Read the model definition and answer for the solid it produces. Units are mm, in the model's axes. A direction names the side the tool comes from. Give positions to 0.01 mm unless a question says otherwise; leave off trailing zeros. Order: outer loops, then holes, each group sorted by start corner. A loop starts at its lowest first (then second) coordinate and runs counter-clockwise, first axis right, second up. Notation, with made-up numbers: (49.25, 29.25) - (89.25, 29.25) arc R27 ccw to (89.25, 66.25) - close; hole circle Ø1 at (27, 53.25). An arc over 180 degrees is marked (long way). Return JSON: item names as keys, results as strings.
```python
from build123d import *

# Parameters (mm, degrees)
F0_R       = 29.175
F1_DEPTH   = 8.35
F1_FACE_R  = 29.175
F3_R       = 15.685
F5_R       = 15.685
F6_DEPTH   = 2.25
F7_R       = 16.25
F8_DEPTH   = 5.75
F9_R       = 29.625
F10_DEPTH  = 14.2
F11_R      = 21
F12_DEPTH  = 8.75
F12_FACE_R = 21
F14_R      = 35
F16_R      = 35
F17_DEPTH  = 10


with BuildPart() as f1:
    # F0 (on Top) → F1 (new body)
    with BuildSketch(Plane.XY):
        Circle(F0_R)
    extrude(amount=F1_DEPTH)

    # F1_face (on face) → F4 section 0
    with BuildSketch(Plane(origin=(0, 0, 0), x_dir=(1, 0, 0), z_dir=(0, 0, -1))):
        Circle(F1_FACE_R)
    # F3 (on offset) → F4 section 1
    with BuildSketch(Plane(origin=(0, 0, -18), x_dir=(1, 0, 0), z_dir=(0, 0, -1))):
        Circle(F3_R)
    loft()

    # F5 (on face) → F6 (join)
    with BuildSketch(Plane(origin=(0, 0, -18), x_dir=(1, 0, 0), z_dir=(0, 0, -1))):
        Circle(F5_R)
    extrude(amount=F6_DEPTH)

    # F7 (on face) → F8 (join)
    with BuildSketch(Plane(origin=(0, 0, -20.25), x_dir=(1, 0, 0), z_dir=(0, 0, -1))):
        Circle(F7_R)
    extrude(amount=F8_DEPTH)

    # F9 (on face) → F10 (join)
    with BuildSketch(Plane(origin=(0, 0, -26), x_dir=(1, 0, 0), z_dir=(0, 0, -1))):
        Circle(F9_R)
    extrude(amount=F10_DEPTH)

    # F11 (on face) → F12 (join)
    with BuildSketch(Plane(origin=(0, 0, -40.2), x_dir=(1, 0, 0), z_dir=(0, 0, -1))):
        Circle(F11_R)
    extrude(amount=F12_DEPTH)

    # F12_face (on face) → F15 section 0
    with BuildSketch(Plane(origin=(0, 0, -48.95), x_dir=(1, 0, 0), z_dir=(0, 0, -1))):
        Circle(F12_FACE_R)
    # F14 (on offset) → F15 section 1
    with BuildSketch(Plane(origin=(0, 0, -63.45), x_dir=(1, 0, 0), z_dir=(0, 0, -1))):
        Circle(F14_R)
    loft()

    # F16 (on face) → F17 (join)
    with BuildSketch(Plane(origin=(0, 0, -63.45), x_dir=(1, 0, 0), z_dir=(0, 0, -1))):
        Circle(F16_R)
    extrude(amount=F17_DEPTH)


solid = f1.part
```
Q1. Consider L1, parallel to Z at x = 3.5, y = 25; L2, parallel to Z at x = -16.5, y = -3; L3, parallel to Z at x = -8.5, y = 14. Determine where each line is inside the solid, lowest interval first.
Values:
{"L1": "z = -73.45 to -53.35, -40.2 to -26, -5.25 to 8.35", "L2": "z = -73.45 to -26, -16.55 to 8.35", "L3": "z = -73.45 to -26, -17.07 to 8.35"}
Q2. Determine the mould class of faces 1 (the conical face through (20.9, -6.6, -49.9)), 2 (the flat face through (0, 0, -73.45)), 3 (the cylindrical face through (-28, 21, -68)), 4 (the flat face through (13, 13, -26)) for opening direction Z: released by +Z, released by -Z, zero draft, split by the parting line, or undercut.
Values:
{"face 1": "undercut", "face 2": "released by -Z", "face 3": "zero draft", "face 4": "undercut"}
Q3. For faces 5 (the flat face through (-16, -1, -20.25)), 6 (the cylindrical face through (-6.325, -28.481, 4.117)), 7 (the flat face through (0, 0, 8.35)), determine the directions among +Z, -Z, +X, -X, +Y, -Y from which every point of the face is accessible in a straight line to the end or side of a thin tool.
Values:
{"face 5": "none", "face 6": "+Z", "face 7": "+Z, +X, -X, +Y, -Y"}
Q4. A cutting plane is placed at C-C (y = 27.5). Give the number of separate pieces and of enclosed holes in the cut face, and give its area (3 significant figures).
Values:
{"separate pieces": "3", "enclosed holes": "0", "area": "1,160 mm²"}
Q5. A cutting plane is placed at B-B (z = -47). Write down the section's boundary in (x, y).
Values:
{"outline": "circle Ø42 at (0, 0)"}
Q6. Given pin 1 (1 mm diameter, centred on x = 6.5, z = -13, fed in from -Y); pin 2 (10 mm diameter, centred on y = 24, z = -62, fed in from +X); pin 3 (8 mm diameter, centred on x = 9.5, z = -27, fed in from +Y), each flat-ended and moving along its own axis, determine where each tip first touches the part or whether it passes through.
Values:
{"pin 1": "stops at y = -18.75", "pin 2": "stops at x = 29.25", "pin 3": "stops at y = 29.11"}
Q7. A cutting plane is placed at A-A (x = 0). Write down the section's boundary in (y, z) (3 decimals).
Values:
{"outline": "(-35, -73.45) - (35, -73.45) - (35, -63.45) - (21, -48.95) - (21, -40.2) - (29.625, -40.2) - (29.625, -26) - (16.25, -26) - (16.25, -20.25) - (15.685, -20.25) - (15.685, -18) - (29.175, 0) - (29.175, 8.35) - (-29.175, 8.35) - (-29.175, 0) - (-15.685, -18) - (-15.685, -20.25) - (-16.25, -20.25) - (-16.25, -26) - (-29.625, -26) - (-29.625, -40.2) - (-21, -40.2) - (-21, -48.95) - (-35, -63.45) - close"}
